Geometry: final body of the model. Coordinates: model frame, mm. A direction names the side the tool comes from. Give positions to 0.01 mm unless a question says otherwise; leave off trailing zeros. Write each loop counter-clockwise with the first axis right and the second up, starting at its lowest first coordinate (ties: lowest second). Pieces come first, ordered by that corner, then holes. Notation, with made-up numbers: M 56,46 L 78,46 A16 ccw 78,64 Z; hole C -31.5,45 d5. An arc over 180 degrees is marked long. Use a Markdown table: item, result. Add a question column.
(1) Cut plane C-C (z = 101). Output: boundary loops of the cut face in (x, y).
(2) Material intervals for L1, parallel to Y at x = 23.5, z = 103.5; L2, parallel to X at y = 55, z = 57.5; L3, parallel to Y at x = 29, z = 93, sorted ascending.
(3) Reachability of faces 1 (the flat face through (13, 62, 0)), 2 (the flat face through (19.9, 69.4, 56.3)) from +Z, -Z, +X, -X, +Y, -Y: full face, straight path, thin tool, end or side. Return the list, or none.
(4) Cut plane A-A (x = 11). Output: boundary loops of the cut face in (y, z), plus the area to 3 significant figures.
(5) Pin query (flat end, axial travel): pin 1 Ø2 at (y, z) = (45.5, 60) entering from +X; pin 2 Ø5 at (y, z) = (37.5, 36.5) entering from -X; pin 3 Ø4 at (x, z) = (4, 39.5) entering from +Y. Return the tip coordinate at first contact, or that it passes through.
(6) Draft query along X for faces 3 (the flat face through (28.4, 69.44, 56.35)), 4 (the cylindrical face through (22.591, -2.035, 56.35)), 5 (the flat face through (13, 62, 114.3)). Return one class per face: released by +X, released by -X, zero draft, split by the parting line, or undercut.
(7) Cut plane B-B (y = 9). Output: boundary loops of the cut face in (x, z), plus the area to 3 significant figures.
```python
from build123d import *

# Parameters (mm, degrees)
F0_R     = 28.872243
F1_DEPTH = 114.3


with BuildPart() as f1:
    # F0 (on Top) → F1 (new body)
    with BuildSketch(Plane.XY):
        with BuildLine():
            ThreePointArc((16.699345, 71.255645), (24.115243, -2.066448), (31.531141, 71.255645))
            Line((31.531141, 71.255645), (25.186695, 67.577745))
            ThreePointArc((25.186695, 67.577745), (24.115243, 67.595343), (23.043791, 67.577745))
            Line((23.043791, 67.577745), (16.699345, 71.255645))
        make_face()
        with Locations((24.115243, 34.969625)):
            Circle(F0_R, mode=Mode.SUBTRACT)
    extrude(amount=F1_DEPTH)


solid = f1.part
```
Answer list:
| question | item | result |
|---|---|---|
| 1 | outline | M 16.7,71.26 A37.04 ccw long 31.53,71.26 L 25.19,67.58 A32.63 ccw 23.04,67.58 Z; hole C 24.12,34.97 d57.74 |
| 2 | L1 | -2.06 to 6.1, 63.84 to 67.59 |
| 2 | L2 | -7.04 to 3.32, 44.91 to 55.27 |
| 2 | L3 | -1.74 to 6.51, 63.43 to 69.79 |
| 3 | face 1 | -Z, +X, -X, +Y, -Y |
| 3 | face 2 | +Z, -Z, +Y |
| 4 | outline | M 0.33,0 L 9.25,0 L 9.25,114.3 L 0.33,114.3 Z; M 60.69,0 L 69.61,0 L 69.61,114.3 L 60.69,114.3 Z |
| 4 | area | 2,040 mm² |
| 5 | pin 1 | x = 59.9 |
| 5 | pin 2 | x = -12.92 |
| 5 | pin 3 | y = 67.27 |
| 6 | face 3 | undercut |
| 6 | face 4 | split by the parting line |
| 6 | face 5 | zero draft |
| 7 | outline | M -2.29,0 L 11.5,0 L 11.5,114.3 L -2.29,114.3 Z; M 36.73,0 L 50.52,0 L 50.52,114.3 L 36.73,114.3 Z |
| 7 | area | 3,150 mm² |
